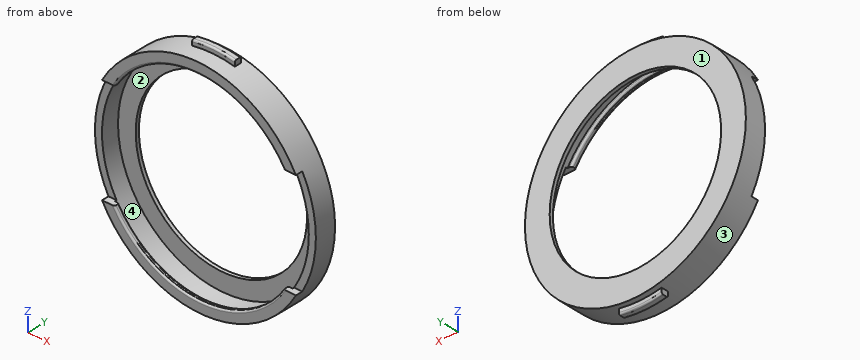
from build123d import *

# Parameters (mm, degrees)
SKETCH1_R                = 31.25
SKETCH1_R_2              = 29.25
BOSS_EXTRUDE2_DEPTH      = 8
SKETCH3_R                = 29.25
SKETCH3_R_2              = 28.25
BOSS_EXTRUDE3_DEPTH      = 1.5
FILLET1_R                = 0.5
SKETCH4_R                = 29.25
SKETCH4_R_2              = 24.25
BOSS_EXTRUDE4_DEPTH      = 1
CUT_EXTRUDE3_START       = 5
SKETCH5_W                = 70
SKETCH5_H                = 30
CUT_EXTRUDE3_DEPTH       = 2
BOSS_EXTRUDE5_DEPTH      = 1
BOSS_EXTRUDE5_DEPTH_BACK = 1
FILLET3_R                = 0.5


with BuildPart() as part:
    # Sketch1 → Boss-Extrude2 (new body)
    with BuildSketch(Plane(origin=(0, 0, 0), x_dir=(1, 0, 0), z_dir=(0, 1, 0))):
        Circle(SKETCH1_R)
        Circle(SKETCH1_R_2, mode=Mode.SUBTRACT)
    extrude(amount=BOSS_EXTRUDE2_DEPTH)

    # Sketch3 → Boss-Extrude3 (add)
    with BuildSketch(Plane(origin=(0, 1.5, 0), x_dir=(1, 0, 0), z_dir=(0, 1, 0))):
        Circle(SKETCH3_R)
        Circle(SKETCH3_R_2, mode=Mode.SUBTRACT)
    extrude(amount=-BOSS_EXTRUDE3_DEPTH)

    # Fillet1
    fillet1_edges = [part.edges().sort_by_distance(p)[0] for p in [
        (-28.25, 0, 0),
        (-28.25, 1.5, 0),
    ]]
    fillet(fillet1_edges, radius=FILLET1_R)

    # Sketch4 → Boss-Extrude4 (add)
    with BuildSketch(Plane(origin=(0, 8, 0), x_dir=(1, 0, 0), z_dir=(0, 1, 0))):
        Circle(SKETCH4_R)
        Circle(SKETCH4_R_2, mode=Mode.SUBTRACT)
    extrude(amount=-BOSS_EXTRUDE4_DEPTH)

    # Sketch5 → Cut-Extrude3 (cut)
    with BuildSketch(Plane.XZ.offset(-7).offset(CUT_EXTRUDE3_START)):
        Rectangle(SKETCH5_W, SKETCH5_H)
    extrude(amount=CUT_EXTRUDE3_DEPTH, mode=Mode.SUBTRACT)

    # Sketch6 → Boss-Extrude5 (add, two sides)
    with BuildSketch(Plane(origin=(0, 5.5, 0), x_dir=(1, 0, 0), z_dir=(0, 1, 0))) as boss_extrude5_sk:
        with BuildLine():
            Line((6.051043417, 30.658561179), (6.051043417, 32.186136357))
            ThreePointArc((6.051043417, 32.186136357), (0, 32.75), (-6.051043417, 32.186136357))
            Line((-6.051043417, 32.186136357), (-6.051043417, 30.658561179))
            ThreePointArc((-6.051043417, 30.658561179), (0, 31.25), (6.051043417, 30.658561179))
        make_face()
        with BuildLine():
            Line((-6.051043417, -32.186136357), (-6.051043417, -30.658561179))
            ThreePointArc((-6.051043417, -30.658561179), (0, -31.25), (6.051043417, -30.658561179))
            Line((6.051043417, -30.658561179), (6.051043417, -32.186136357))
            ThreePointArc((6.051043417, -32.186136357), (0, -32.75), (-6.051043417, -32.186136357))
        make_face()
    extrude(amount=BOSS_EXTRUDE5_DEPTH)
    extrude(boss_extrude5_sk.sketch, amount=-BOSS_EXTRUDE5_DEPTH_BACK)

    # Fillet3
    fillet3_edges = [part.edges().sort_by_distance(p)[0] for p in [
        (0, 4.5, -32.75),
        (0, 6.5, -32.75),
        (0, 4.5, 32.75),
        (0, 6.5, 32.75),
    ]]
    fillet(fillet3_edges, radius=FILLET3_R)


solid = part.part
Read the model definition and answer for the solid it produces. Units are mm, in the model's axes. Face numbers are marked on the shaded views. Give positions to 0.01 mm unless a question says otherwise; leave off trailing zeros. Write each loop counter-clockwise with the first axis right and the second up, starting at its lowest first coordinate (ties: lowest second). Pieces come first, ordered by that corner, then holes. Notation, with made-up numbers: (75, -36) - (130, -36) arc R29 cw to (130, -5) - close; hole circle Ø6 at (12, 26.25). An arc over 180 degrees is marked (long way). Return JSON: item names as keys, results as strings.
Q1. A cutting plane is placed at C-C, the plane y = 3.75. Determine the outline of the cut face in (x, z).
Reply:
{"outline": "circle Ø62.5 at (0, 0); hole circle Ø58.5 at (0, 0)"}
Q2. Consider line 1 along X through (y, z) = (4.85, 0); line 2 along Z through (x, y) = (0, 7.5); line 3 along Z through (x, y) = (0, 5.1). Determine where each line is inside the solid, lowest interval first. Write a range as [from, to].
Reply:
{"line 1": "[-31.25, -29.25], [29.25, 31.25]", "line 2": "[-31.25, -24.25], [24.25, 31.25]", "line 3": "[-32.75, -29.25], [29.25, 32.75]"}
Q3. A cutting plane is placed at D-D, the plane x = 26. Determine the outline of the cut face in (y, z).
Reply:
{"outline": "(0, -17.34) - (8, -17.34) - (8, 17.34) - (0, 17.34) - (0, 15) - (2, 15) - (2, 13.4) - (7, 13.4) - (7, -13.4) - (2, -13.4) - (2, -15) - (0, -15) - close"}
Q4. For a pull along X with two mould halves and no side action, classify the marked faces 1, 2, 3 and 4 as released by +X, released by -X, zero draft, split by the parting line, or undercut.
Reply:
{"face 1": "zero draft", "face 2": "undercut", "face 3": "split by the parting line", "face 4": "undercut"}
Q5. Given P1, Ø3, axis at x = 29, z = 4.5, coming from the -Y side; P2, Ø1.2, axis at y = 6, z = 31.5, coming from the +X side; P3, Ø2, axis at x = -26, y = 1, coming from the -Z side, each flat-ended and moving along its own axis, determine where each tip first touches the part or whether it passes through.
Reply:
{"P1": "y = 2", "P2": "x = 6.05", "P3": "z = -18.75"}
Q6. A cutting plane is placed at B-B, the plane z = 0. Determine the outline of the cut face in (x, y), and give its area (3 significant figures).
Reply:
{"outline": "(-31.25, 2) - (-29.25, 2) - (-29.25, 7) - (-24.25, 7) - (-24.25, 8) - (-31.25, 8) - close; (24.25, 7) - (29.25, 7) - (29.25, 2) - (31.25, 2) - (31.25, 8) - (24.25, 8) - close", "area": "34.0 mm²"}
